from build123d import *

# Parameters (mm, degrees)
SKETCH1_R           = 4.7625
BOSS_EXTRUDE1_DEPTH = 14.3002
SKETCH2_R           = 1.5875
CUT_EXTRUDE1_DEPTH  = 15.3002
SKETCH2_3_R         = 3.175
SKETCH2_3_R_2       = 1.5875
CUT_EXTRUDE2_DEPTH  = 6.35
SKETCH4_R           = 1.3589
CUT_EXTRUDE3_DEPTH  = 10.525


with BuildPart() as part:
    # Sketch1 → Boss-Extrude1 (new body)
    with BuildSketch(Plane.XY):
        Circle(SKETCH1_R)
    extrude(amount=BOSS_EXTRUDE1_DEPTH)

    # Sketch2 → Cut-Extrude1 (cut, through all)
    with BuildSketch(Plane(origin=(0, 0, 0), x_dir=(-1, 0, 0), z_dir=(0, 0, -1))):
        Circle(SKETCH2_R)
    extrude(amount=-CUT_EXTRUDE1_DEPTH, mode=Mode.SUBTRACT)

    # Sketch2<3> → Cut-Extrude2 (cut)
    with BuildSketch(Plane(origin=(0, 0, 0), x_dir=(-1, 0, 0), z_dir=(0, 0, -1))):
        Circle(SKETCH2_3_R)
        Circle(SKETCH2_3_R_2, mode=Mode.SUBTRACT)
    extrude(amount=-CUT_EXTRUDE2_DEPTH, mode=Mode.SUBTRACT)

    # Sketch4 → Cut-Extrude3 (cut, through all)
    with BuildSketch(Plane(origin=(0, 4.7625, 0), x_dir=(1, 0, 0), z_dir=(0, 1, 0))):
        with Locations((0, -10.3124)):
            Circle(SKETCH4_R)
    extrude(amount=-CUT_EXTRUDE3_DEPTH, mode=Mode.SUBTRACT)


solid = part.part
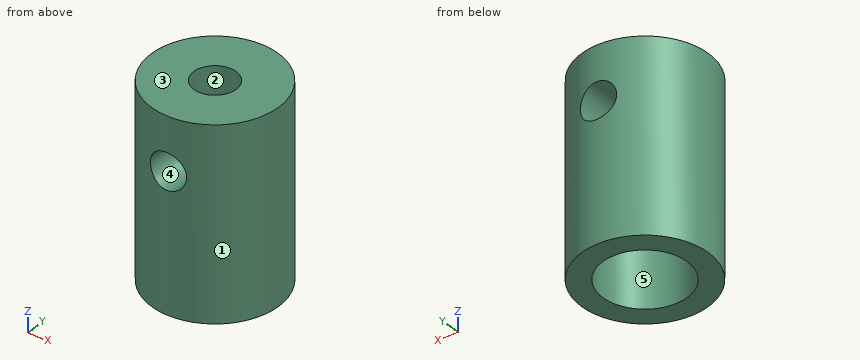
Source: CAD feature listing. Evaluate the final solid. Frame: model axes, mm. Face numbers are marked on the shaded views. A direction names the side the tool comes from. Round coordinates to 2 decimals unless told otherwise and drop trailing zeros. Order: outer loops, then holes, each group sorted by start corner. A loop starts at its lowest first (then second) coordinate and runs counter-clockwise, first axis right, second up. Notation, with made-up numbers: (38.25, 18) - (88.25, 18) arc R19 cw to (88.25, 36) - close; hole circle Ø11 at (86.25, 8). An arc over 180 degrees is marked (long way). Use a Markdown table: item, result. Add a question column.
1. Mould query, pull axis Y, two halves, no side actions, for the marked faces 1, 2 and 3. Classes: +Y half, -Y half, draft (parallel to the pull), parting line (faces both ways), or undercut.
2. Line query: probe 1 along Z at (x, y) = (0, -3.3); probe 2 along Y at (x, z) = (0, 1.5) (1 decimal); probe 3 along Z at (x, y) = (-2, 0.25). Output: solid intervals per line, ascending.
3. First-contact query: pin 1 (2 mm diameter, centred on x = 2.5, z = 12.5, fed in from -Y); pin 2 (2.5 mm diameter, centred on x = 0, z = 10.31, fed in from -Y); pin 3 (5.5 mm diameter, centred on x = 0, y = 0, fed in from -Z). Flat tips, straight axial feed; report the tip coordinate or a pass-through.
4. Set-up query: the marked faces 4 and 5. Return all of +Z, -Z, +X, -X, +Y, -Y with unobstructed straight access to the full face (end or side cutting, diameter ignored); none if empty.
5. Section query A-A (x = 0). Give the number of separate pieces and of enclosed holes in the cut face, then the cut area to 3 significant figures.
6. Section query D-D (z = 9.75). Return the cut outline in (x, y) (1 decimal), then the cut area to 3 significant figures.
Derived:
| question | item | result |
|---|---|---|
| 1 | face 1 | parting line |
| 1 | face 2 | undercut |
| 1 | face 3 | draft |
| 2 | probe 1 | 0 to 8.95, 11.67 to 14.3 |
| 2 | probe 2 | -4.8 to -3.2, 3.2 to 4.8 |
| 2 | probe 3 | 6.35 to 14.3 |
| 3 | pin 1 | y = -4.52 |
| 3 | pin 2 | through |
| 3 | pin 3 | z = 6.35 |
| 4 | face 4 | +Y, -Y |
| 4 | face 5 | -Z |
| 5 | separate pieces | 4 |
| 5 | enclosed holes | 0 |
| 5 | area | 53.4 mm2 |
| 6 | outline | (-1.2, -4.6) - (-1.2, -1) arc R1.6 cw to (-1.2, 1) - (-1.2, 4.6) arc R4.8 ccw to start; (1.2, -4.6) arc R4.8 ccw to (1.2, 4.6) - (1.2, 1) arc R1.6 cw to (1.2, -1) - close |
| 6 | area | 47.0 mm2 |
